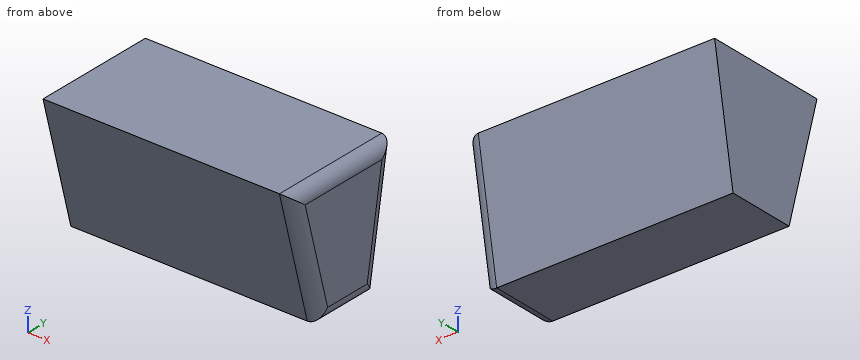
from build123d import *

# Parameters (mm, degrees)
F1_DEPTH = 101.6
F2_R     = 5.08


with BuildPart() as f1:
    # F0 (on Right) → F1 (new body)
    with BuildSketch(Plane.YZ):
        Polygon((27.6941948846, 46.3221500594), (-23.1058051154, 46.3221500594), (-9.271863848, -5.6394003332), (18.5437425971, -5.6394003332), align=None)
    extrude(amount=F1_DEPTH)

    # F2
    f2_edges = [f1.edges().sort_by_distance(p)[0] for p in [
        (101.6, -16.188834, 20.341375),
        (101.6, 4.635939, -5.6394),
        (101.6, 23.118969, 20.341375),
        (101.6, 2.294195, 46.32215),
    ]]
    fillet(f2_edges, radius=F2_R)


solid = f1.part
Design review of the part built by this model. Coordinates are the model's own, in mm. Coordinates: 2 decimals unless noted, no trailing zeros. Order: outer loops, then holes, each group sorted by start corner. A loop starts at its lowest first (then second) coordinate and runs counter-clockwise, first axis right, second up.
Item 1: Take a section at A-A, the plane x = 51. Write out the cut boundary in (y, z).
Item 2: For line 1 (X direction, y = 19.5, z = 27); line 2 (Y direction, x = 41.5, z = 41); line 3 (Y direction, x = 23.5, z = 10.5), list the stretches that pass through material, from the lowest coordinate up.
Item 3: For pin 1 Ø6 at (x, z) = (37, 11.5) entering from +Y; pin 2 Ø1.5 at (x, z) = (16, 33) entering from -Y; pin 3 Ø6 at (x, z) = (75.5, 22) entering from +Y, all flat-tipped, find the tip position at first contact; note any pin that passes through.
The answers:
1. outline: (-23.11, 46.32) - (-9.27, -5.64) - (18.54, -5.64) - (27.69, 46.32) - close
2. line 1: x = 0 to 101.59
2. line 2: y = -21.69 to 26.76
2. line 3: y = -13.57 to 21.39
3. pin 1: stops at y = 22.09
3. pin 2: stops at y = -19.76
3. pin 3: stops at y = 23.94
